Part model, mm, in its own coordinate system. A direction names the side the tool comes from. Round coordinates to 2 decimals unless told otherwise and drop trailing zeros. Write each loop counter-clockwise with the first axis right and the second up, starting at its lowest first coordinate (ties: lowest second). Pieces come first, ordered by that corner, then holes. Notation, with made-up numbers: M 73.5,77.25 L 78.5,77.25 A31 ccw 78.5,103.25 Z; hole C -3.75,82 d7. An arc over 180 degrees is marked long. Use a Markdown table: item, result. Add a question column.
1) Drop flat-ended pins along their axis: P1, Ø7, axis at x = 0, z = 0, coming from the +Y side; P2, Ø10.5, axis at x = 0, z = -100, coming from the -Y side; P3, Ø4, axis at x = 0, z = -170, coming from the +Y side. Give the stop position or say it passes through.
2) Slice it at C-C on z = -21. Write the cut outline in (x, y), plus the area to 3 significant figures.
3) Slice it at A-A on z = -130. Write the cut outline in (x, y).
4) Two-plate mould, pull along Z, no slides. Class faces 3 (the face through (-0.98, 0.49, -134.39)), 4 (the face through (2, 10, -5)), 5 (the face through (-1.302, 6.041, 9.915)): released by +Z, released by -Z, zero draft, split by the parting line, or undercut.
5) Which spindle directions (+Z, -Z, +X, -X, +Y, -Y) get a long thin tool onto all of the face, cutting with end or side? Do faces 1 (the face through (-0.59, 0.49, -110.54)), 2 (the face through (1.08, 2.97, -95.12)). Say none if no direction does.
6) Slice it at B-B on y = 3.5. Write the cut outline in (x, z), plus the area to 3 significant figures.
7) Wall check: probe 1 along X at (y, z) = (2.5, -99.5); probe 2 along X at (y, z) = (1.3, -170); probe 3 along Y at (x, z) = (-1, -154). Give the ranges that are in metal, low to high.
Autodesk Inventor part; units mm, degrees
ref_plane "YZ Plane" through (0, 0, 0) normal (1, 0, 0) x (0, 1, 0)
ref_plane "XZ Plane" through (0, 0, 0) normal (0, 1, 0) x (-1, 0, 0)
ref_plane "XY Plane" through (0, 0, 0) normal (0, 0, 1) x (1, 0, 0)
sketch "Skizze3" plane through (0, 0, 0) normal (0, 1, 0) x (-1, 0, 0)
  line L0 (0, 0) -> (0, -180) construction
  line L1 (-10, 0) -> (-10, -180)
  line L2 (10, -180) -> (10, 0)
  arc A0 (10, 0) -> (-10, 0) centre (0, 0) ccw
  arc A1 (-10, -180) -> (10, -180) centre (0, -180) ccw
  circle A2 centre (0, 0) radius 5
  circle A3 centre (0, -180) radius 5
  circle A4 centre (0, -170) radius 1.5
  circle A5 centre (0, -130) radius 5
  circle A6 centre (0, -115) radius 5
  circle A7 centre (0, -100) radius 5
  circle A8 centre (0, 0) radius 4.5
  point P0 (0, -90)
  dimension "d4" = 180
  dimension "d5" = 10
  dimension "d6" = 10
  dimension "d7" = 10
  dimension "d8" = 3
  dimension "d9" = 10
  dimension "d10" = 50
  dimension "d11" = 10
  dimension "d12" = 10
  dimension "d13" = 10
  dimension "d14" = 15
  dimension "d15" = 15
  dimension "d27" = 9
extrude "Extrusion3" add sketch "Skizze3" along normal blind 5 contours A0 L2 A1 L1
sketch "Skizze4" plane through (0, 5, 0) normal (0, 1, 0) x (1, 0, 0)
  circle A0 centre (0, 0) radius 5
  circle A1 centre (0, 0) radius 10
  dimension "d18" = 20
extrude "Extrusion4" add sketch "Skizze4" along normal blind 5
extrude "Extrusion5" add sketch "Skizze3" along normal blind 6 contours A2
sketch "Skizze5" plane through (0, 0, 0) normal (0, -1, 0) x (1, 0, 0)
  circle A0 centre (0, -130) radius 5
  circle A1 centre (0, -100) radius 5
  circle A2 centre (0, -115) radius 5
  circle A3 centre (0, -100) radius 4.5
  circle A4 centre (0, -115) radius 4.5
  circle A5 centre (0, -130) radius 4.5
  point P0 (0, 0)
  dimension "d28" = 9
  dimension "d29" = 9
  dimension "d30" = 9
extrude "Extrusion7" add sketch "Skizze5" against normal blind 1
properties part number "BT303_trajan20_21" material "Kunststoff, undurchsichtig Schwarz"
Entries:
| question | item | result |
|---|---|---|
| 1 | P1 | passes through |
| 1 | P2 | stops at y = 0 |
| 1 | P3 | stops at y = 5 |
| 2 | outline | M -10,0 L 10,0 L 10,5 L -10,5 Z |
| 2 | area | 100 mm^2 |
| 3 | outline | M -10,0 L -4.5,0 L -4.5,1 L -5,1 L -5,5 L -10,5 Z; M 4.5,0 L 10,0 L 10,5 L 5,5 L 5,1 L 4.5,1 Z |
| 4 | face 3 | undercut |
| 4 | face 4 | zero draft |
| 4 | face 5 | split by the parting line |
| 5 | face 1 | +Y, -Y |
| 5 | face 2 | +Y |
| 6 | outline | M -10,-180 A10 ccw 10,-180 L 10,0 A10 ccw -10,0 Z; hole C 0,-180 d10; hole C 0,-130 d10; hole C 0,-115 d10; hole C 0,-100 d10; hole C 0,0 d9; hole C 0,-170 d3 |
| 6 | area | 3,530 mm^2 |
| 7 | probe 1 | x = -10 to -4.97, 4.97 to 10 |
| 7 | probe 2 | x = -10 to -1.5, 1.5 to 10 |
| 7 | probe 3 | y = 0 to 5 |
